CAD build for the part. Positions are in the model's coordinates, mm. A direction names the side the tool comes from. Round coordinates to 2 decimals unless told otherwise and drop trailing zeros. Order: outer loops, then holes, each group sorted by start corner. A loop starts at its lowest first (then second) coordinate and runs counter-clockwise, first axis right, second up.
```python
from build123d import *

# Parameters (mm, degrees)
SKETCH1_R           = 6.35
BOSS_EXTRUDE1_DEPTH = 12.7
SKETCH1_3_R         = 3.175
BOSS_EXTRUDE2_DEPTH = 6.35
SKETCH1_4_R         = 3.175
BOSS_EXTRUDE3_DEPTH = 99.06


with BuildPart() as part:
    # Sketch1 → Boss-Extrude1 (new body)
    with BuildSketch(Plane.XY):
        Circle(SKETCH1_R)
    extrude(amount=-BOSS_EXTRUDE1_DEPTH)

    # Sketch1<3> → Boss-Extrude2 (add)
    with BuildSketch(Plane.XY):
        with BuildLine():
            Line((9.510289567, -57.679166667), (12.680386089, -0.705555556))
            ThreePointArc((12.680386089, -0.705555556), (0, 12.7), (-12.680386089, -0.705555556))
            Line((-12.680386089, -0.705555556), (-9.510289567, -57.679166667))
            ThreePointArc((-9.510289567, -57.679166667), (0, -66.675), (9.510289567, -57.679166667))
        make_face()
        with Locations((0, -57.15)):
            Circle(SKETCH1_3_R, mode=Mode.SUBTRACT)
    extrude(amount=BOSS_EXTRUDE2_DEPTH)

    # Sketch1<4> → Boss-Extrude3 (add)
    with BuildSketch(Plane.XY):
        with Locations((0, -57.15)):
            Circle(SKETCH1_4_R)
    extrude(amount=BOSS_EXTRUDE3_DEPTH)


solid = part.part
```
1. Cut at B-B, the plane z = 47. Write the cut outline in (x, y) (3 decimals), and give its area (3 significant figures).
2. Pin check, flat tips, straight feed: P1, Ø4, axis at x = -1.5, z = -1.5, coming from the -Y side; P2, Ø12, axis at x = -7.5, y = 2, coming from the +Z side; P3, Ø7.5, axis at x = -6, y = -10, coming from the -Z side. Stop position of each tip, or through.
3. Cut at D-D, the plane z = 4. Write the cut outline in (x, y) (3 decimals), and give its area (3 significant figures).
4. Drill centre lines: line 1 (Z direction, x = 3, y = -26.5); line 2 (Z direction, x = -0.25, y = 6); line 3 (Y direction, x = 3.25, z = 0.5). Where is each one in solid material? Low to high.
5. Tool access for faces 1 (the face through (1.707, -54.473, 52.056)), 2 (the face through (0, 0, -12.7)), 3 (the face through (-1.38, -6.2, -6.26)): list every direction of +Z, -Z, +X, -X, +Y, -Y with a clear straight run to the whole face (end or side of a thin tool).
6. Cut at A-A, the plane x = 0. Write the cut outline in (y, z) (3 decimals), and give its area (3 significant figures).
7. Cut at C-C, the plane y = -37.5. Write the cut outline in (x, z).
Outcome:
1. outline: circle Ø6.35 at (0, -57.15)
1. area: 31.7 mm2
2. P1: stops at y = -66.67
2. P2: stops at z = 6.35
2. P3: stops at z = 0
3. outline: (-12.68, -0.706) - (-9.51, -57.679) arc R9.525 ccw to (9.51, -57.679) - (12.68, -0.706) arc R12.7 ccw (long way) to start
3. area: 1,670 mm2
4. line 1: z = 0 to 6.35
4. line 2: z = -12.7 to 6.35
4. line 3: y = -66.1 to 12.28
5. face 1: +Z
5. face 2: -Z, +X, -X, +Y, -Y
5. face 3: -Z
6. outline: (-66.675, 0) - (-6.35, 0) - (-6.35, -12.7) - (6.35, -12.7) - (6.35, 0) - (12.7, 0) - (12.7, 6.35) - (-53.975, 6.35) - (-53.975, 99.06) - (-60.325, 99.06) - (-60.325, 6.35) - (-66.675, 6.35) - close
6. area: 1,250 mm2
7. outline: (-10.63, 0) - (10.63, 0) - (10.63, 6.35) - (-10.63, 6.35) - close
